Work out the finished part from the listing and answer in its coordinate system (mm). A direction names the side the tool comes from. Coordinates: 2 decimals unless noted, no trailing zeros. Write each loop counter-clockwise with the first axis right and the second up, starting at its lowest first coordinate (ties: lowest second). Pieces come first, ordered by that corner, then holes. Notation, with made-up numbers: (51.5, 82.5) - (64.5, 82.5) arc R27 cw to (64.5, 98.5) - close; hole circle Ø7 at (70.5, 11.25). An arc over 180 degrees is marked (long way). Use a Markdown table: item, result. Add a question column.
(1) The part is cut by section B-B, the plane y = 0. Give the vertices of the cut face in (x, z), then the cut area to 3 significant figures.
(2) The part is cut by section D-D, the plane z = 1.75. Give the vertices of the cut face in (x, y).
(3) Given pin 1 Ø3 at (x, y) = (-1, 3) entering from +Z; pin 2 Ø2.5 at (y, z) = (-2, 1.5) entering from -X; pin 3 Ø4 at (x, z) = (-1.5, 2.5) entering from +Y, each flat-ended and moving along its own axis, determine where each tip first touches the part or whether it passes through.
(4) A tool of negligible diameter and unlimited length cuts with its end or side. For faces 1 (the face through (0, -10, 0)), 2 (the face through (0, -7, 2)), 3 (the face through (4, -2, -4.5)), 4 (the face through (6, -14.95, -4)), from which of +Z, -Z, +X, -X, +Y, -Y can it reach the whole face along a straight path? Write none if from no direction.
(5) The part is cut by section C-C, the plane x = 0. Give the vertices of the cut face in (y, z).
(6) Find the intervals of material crossed by line 1 (Y direction, x = 0, z = -1.9); line 2 (Z direction, x = 0.75, y = 4); line 3 (X direction, y = -6.5, z = 4.25), in increasing order. Write a range as from..to.
(7) The part is cut by section A-A, the plane z = -3. Give the vertices of the cut face in (x, y).
from build123d import *

# Parameters (mm, degrees)
F0_W     = 10
F0_H     = 14
F0_R     = 3.5
F1_DEPTH = 4.5
F2_DEPTH = 5
F4_DEPTH = 25


with BuildPart() as f1:
    # F0 (on Top) → F1 (new body)
    with BuildSketch(Plane.XY):
        Polygon((8, 7), (5, 7), (5, -7), (-5, -7), (-5, -10), (5, -10), (5, -18), (8, -18), align=None)
        Rectangle(F0_W, F0_H)
        Circle(F0_R, mode=Mode.SUBTRACT)
    extrude(amount=-F1_DEPTH)

    # F0 (on Top) → F2 (join)
    with BuildSketch(Plane.XY):
        Polygon((8, 7), (5, 7), (5, -7), (-5, -7), (-5, -10), (5, -10), (5, -18), (8, -18), align=None)
    extrude(amount=F2_DEPTH)

    # F3 (on face) → F4 (cut)
    with BuildSketch(Plane(origin=(5, 0, 0), x_dir=(0, -1, 0), z_dir=(-1, 0, 0))):
        with BuildLine():
            Line((14.95, -4.5), (14.95, -2.5))
            ThreePointArc((14.95, -2.5), (13.3, -4.15), (11.65, -2.5))
            Line((11.65, -2.5), (11.65, -4.5))
            Line((11.65, -4.5), (14.95, -4.5))
        make_face()
        with BuildLine():
            ThreePointArc((11.65, -2.5), (13.3, -4.15), (14.95, -2.5))
            ThreePointArc((14.95, -2.5), (13.3, -0.85), (11.65, -2.5))
        make_face()
    extrude(amount=-F4_DEPTH, mode=Mode.SUBTRACT)


solid = f1.part
Model answer:
| question | item | result |
|---|---|---|
| 1 | outline | (-5, -4.5) - (-3.5, -4.5) - (-3.5, 0) - (-5, 0) - close; (3.5, -4.5) - (8, -4.5) - (8, 5) - (5, 5) - (5, 0) - (3.5, 0) - close |
| 1 | area | 42.0 mm^2 |
| 2 | outline | (-5, -10) - (5, -10) - (5, -18) - (8, -18) - (8, 7) - (5, 7) - (5, -7) - (-5, -7) - close |
| 3 | pin 1 | z = 0 |
| 3 | pin 2 | x = 5 |
| 3 | pin 3 | y = -7 |
| 4 | face 1 | +Z, -Z, -X, -Y |
| 4 | face 2 | +Z, -X, +Y |
| 4 | face 3 | -Z, +X, -X, +Y, -Y |
| 4 | face 4 | -Z, +X, -X |
| 5 | outline | (-10, -4.5) - (-3.5, -4.5) - (-3.5, 0) - (-7, 0) - (-7, 5) - (-10, 5) - close; (3.5, -4.5) - (7, -4.5) - (7, 0) - (3.5, 0) - close |
| 6 | line 1 | -10..-3.5, 3.5..7 |
| 6 | line 2 | -4.5..0 |
| 6 | line 3 | 5..8 |
| 7 | outline | (-5, -10) - (5, -10) - (5, -11.65) - (8, -11.65) - (8, 7) - (-5, 7) - close; (5, -18) - (8, -18) - (8, -14.95) - (5, -14.95) - close; hole circle Ø7 at (0, 0) |
